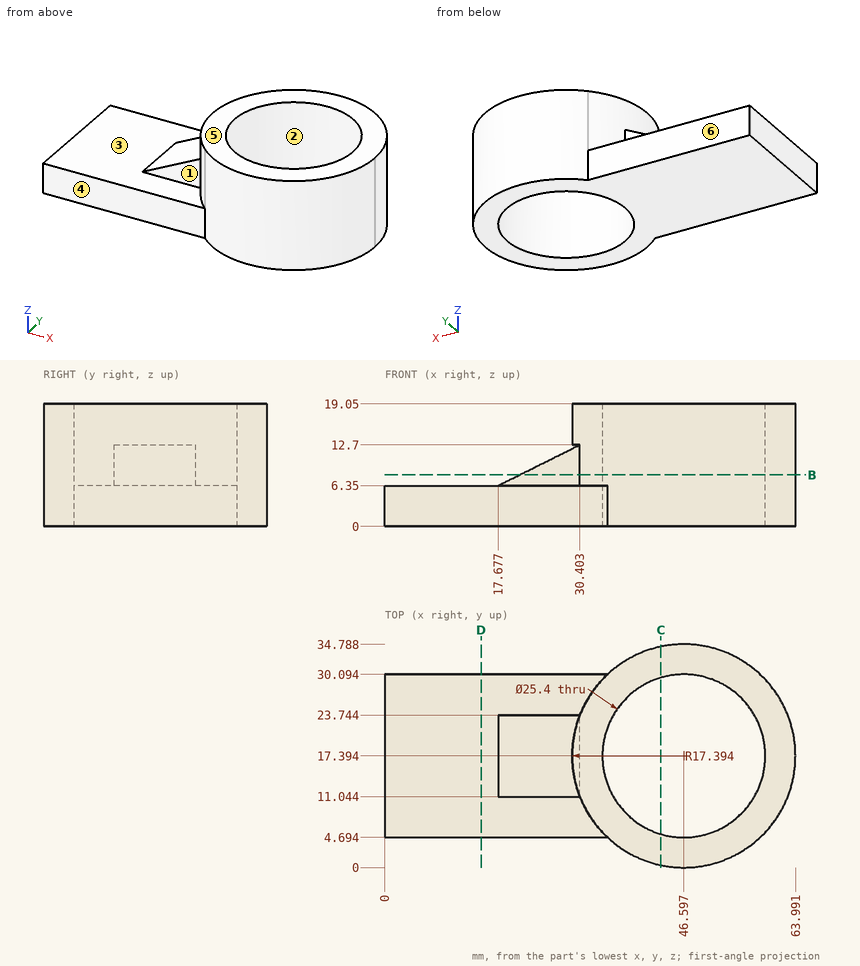
The drawing under review shows one solid part. Ordinate dimensions are in mm from its lowest x, y, z. A direction names the side the tool comes from. Coordinates: 2 decimals unless noted, no trailing zeros. Write each loop counter-clockwise with the first axis right and the second up, starting at its lowest first coordinate (ties: lowest second). Pieces come first, ordered by that corner, then holes. Notation, with made-up numbers: (41, 42.5) -> (53, 42.5) arc R36 cw to (53, 80.5) -> close; hole circle Ø4 at (56, -27.5). An arc over 180 degrees is marked (long way). Write each question's results on one line, items separated by ' | '. Start each with the question number.
1) For the marked faces 4, 5 and 6, list the 3-axis set-ups (+Z, -Z, +X, -X, +Y, -Y) from which the entire face can be reached by the end or side of a thin tool; tool diameter is ignored.
2) The part is to be moulded in two halves that separate along Y. For the marked faces 1, 2 and 3, say which applies: +Y half, -Y half, draft (parallel to the pull), parting line (faces both ways), or undercut.
3) Consider section D-D (x = 15). Write out the cut boundary in (y, z), plus the area to 3 significant figures.
4) Consider section C-C (x = 43). Write out the cut boundary in (y, z).
5) Consider section B-B (z = 8). Write out the cut boundary in (x, y).
6) Insertion check: pin 1 (3 mm diameter, centred on x = 43.5, y = 30, fed in from -Z); pin 2 (6 mm diameter, centred on y = 10, z = 3.5, fed in from +X); pin 3 (3 mm diameter, centred on x = 25, z = 10, fed in from +Y); pin 4 (7 mm diameter, centred on x = 13.5, z = 4.5, fed in from -Y). Each pin has a flat end and moves straight along its axis. Give the tip position at first contact, or say it passes through.
7) Wall thickness on L1, parallel to X at y = 18, z = 13.75; L2, parallel to Y at x = 50.5, z = 1 (1 decimal); L3, parallel to X at y = 21.5, z = 12.75 (1 decimal): over which ranges is each line inside the solid? List them lowest first. Write a range as [from, to].
Geometry says:
1) face 4: +Z, -Z, -X, -Y | face 5: +Z, +X, -X, +Y, -Y | face 6: +Z, -Z, -X, +Y
2) face 1: -Y half | face 2: undercut | face 3: draft
3) outline: (4.69, 0) -> (30.09, 0) -> (30.09, 6.35) -> (4.69, 6.35) -> close | area: 161 mm^2
4) outline: (0.38, 0) -> (5.21, 0) -> (5.21, 19.05) -> (0.38, 19.05) -> close; (29.57, 0) -> (34.41, 0) -> (34.41, 19.05) -> (29.57, 19.05) -> close
5) outline: (20.98, 11.04) -> (30.4, 11.04) arc R17.39 ccw (long way) to (30.4, 23.74) -> (20.98, 23.74) -> close; hole circle Ø25.4 at (46.6, 17.39)
6) pin 1: z = 0 | pin 2: x = 63.43 | pin 3: y = 23.74 | pin 4: y = 4.69
7) L1: [29.21, 33.91], [59.28, 63.98] | L2: [0.4, 5.3], [29.5, 34.3] | L3: [29.7, 34.6], [58.6, 63.5]
